from build123d import *

# Parameters (mm, degrees)
SKETCH1_R           = 3.175
BOSS_EXTRUDE1_DEPTH = 6.096
CUT_EXTRUDE1_DEPTH  = 8.636
SKETCH4_W           = 6.223
SKETCH4_H           = 7.62
CUT_EXTRUDE2_DEPTH  = 81.243500547
SKETCH5_R           = 1.651
CUT_EXTRUDE4_DEPTH  = 6.096


with BuildPart() as part:
    # Sketch1 → Boss-Extrude1 (new body)
    with BuildSketch(Plane.XY):
        Polygon((0, 0), (-38.1, 0), (-38.1, -7.62), (-31.877, -7.62), (-31.877, -15.24), (-38.1, -15.24), (-38.1, -22.86), (-31.877, -22.86), (-31.877, -30.48), (-38.1, -30.48), (-38.1, -38.1), (-31.877, -38.1), (-31.877, -45.72), (-38.1, -45.72), (-38.1, -70.358), (0, -50.8), align=None)
        with Locations(Location((-8.382, -8.382, 0), (0, 0, 180))):
            Circle(SKETCH1_R, mode=Mode.SUBTRACT)
    extrude(amount=BOSS_EXTRUDE1_DEPTH)

    # Sketch2 → Cut-Extrude1 (cut)
    with BuildSketch(Plane(origin=(0, 0, 0), x_dir=(-1, 0, 0), z_dir=(0, 0, -1))):
        Polygon((38.1, 0), (12.7, 0), (38.1, -3.81), align=None)
    extrude(amount=-CUT_EXTRUDE1_DEPTH, mode=Mode.SUBTRACT)

    # Sketch4 → Cut-Extrude2 (cut, through all)
    with BuildSketch(Plane.XY.offset(6.096)):
        with Locations((-34.9885, -57.15)):
            Rectangle(SKETCH4_W, SKETCH4_H)
    extrude(amount=-CUT_EXTRUDE2_DEPTH, mode=Mode.SUBTRACT)

    # Sketch5 → Cut-Extrude4 (cut)
    with BuildSketch(Plane(origin=(0, 0, 0), x_dir=(-1, 0, 0), z_dir=(0, 0, -1))):
        with Locations((9.318987701, -29.697415784)):
            Circle(SKETCH5_R)
    extrude(amount=-CUT_EXTRUDE4_DEPTH, mode=Mode.SUBTRACT)


solid = part.part
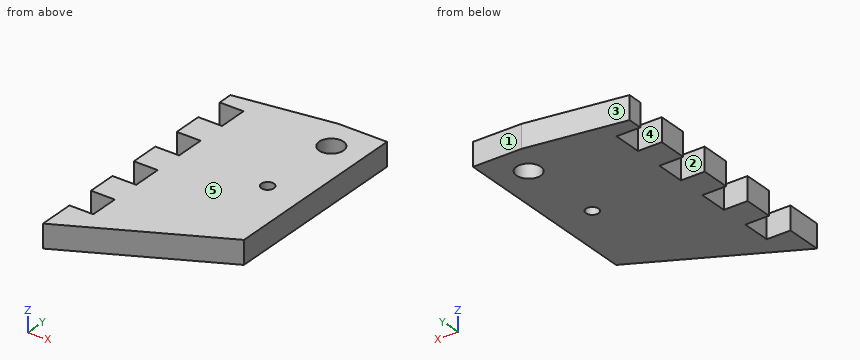
Input: part model. Units: mm. Frame: model coordinates. Face numbers are marked on the shaded views. A direction names the side the tool comes from. Give positions to 0.01 mm unless a question says otherwise; leave off trailing zeros. Write each loop counter-clockwise with the first axis right and the second up, starting at its lowest first coordinate (ties: lowest second). Pieces come first, ordered by that corner, then holes. Notation, with made-up numbers: M 35,65.25 L 70,65.25 A18 ccw 70,90.25 Z; hole C 47.5,27.5 d3. An arc over 180 degrees is marked long. Write item = value, one per line. Start each with the question number.
1) Cut plane C-C on y = -39. Return the cut outline in (x, z), then the cut area to 3 significant figures.
2) Cut plane B-B on z = 3.75. Return the cut outline in (x, y) (3 decimals).
3) Cut plane D-D on x = -3. Return the cut outline in (y, z).
4) Cut plane A-A on x = -7. Return the cut outline in (y, z), then the cut area to 3 significant figures.
5) Reachability of the marked faces 1 and 2 from +Z, -Z, +X, -X, +Y, -Y: full face, straight path, thin tool, end or side. Return the list, or none.
6) First-contact query: pin 1 Ø1.8 at (y, z) = (-28.5, 2.5) entering from -X; pin 2 Ø1.5 at (x, z) = (-22, 4.5) entering from -Y; pin 3 Ø3 at (x, z) = (-36, 3.5) entering from +Y. Flat tips, straight axial feed; report the tip coordinate or a pass-through.
7) Draft query along Y for the marked faces 3, 4 and 5. Return one class per face: +Y half, -Y half, draft (parallel to the pull), parting line (faces both ways), or undercut.
8) Material intervals for line 1 along Y through (x, z) = (-33, 0.5) (3 decimals); line 2 along Y through (x, z) = (-32, 3) (3 decimals); line 3 along X through (y, z) = (-42, 1), sorted ascending. Write a range as [from, to].
Solved:
q1.outline = M -31.88,0 L 0,0 L 0,6.1 L -31.88,6.1 Z
q1.area = 194 mm2
q2.outline = M -38.1,-70.358 L 0,-50.8 L 0,0 L -12.7,0 L -38.1,-3.81 L -38.1,-7.62 L -31.877,-7.62 L -31.877,-15.24 L -38.1,-15.24 L -38.1,-22.86 L -31.877,-22.86 L -31.877,-30.48 L -38.1,-30.48 L -38.1,-38.1 L -31.877,-38.1 L -31.877,-45.72 L -38.1,-45.72 L -38.1,-53.34 L -31.877,-53.34 L -31.877,-60.96 L -38.1,-60.96 Z; hole C -8.382,-8.382 d6.35; hole C -9.319,-29.697 d3.302
q3.outline = M -52.34,0 L 0,0 L 0,6.1 L -52.34,6.1 Z
q4.outline = M -54.39,0 L -11.24,0 L -11.24,6.1 L -54.39,6.1 Z; M -5.52,0 L 0,0 L 0,6.1 L -5.52,6.1 Z
q4.area = 297 mm2
q5.face_1 = +Z, -Z, +X, -X, +Y
q5.face_2 = +Z, -Z, -X
q6.pin_1 = -31.88
q6.pin_2 = -62.48
q6.pin_3 = -3.27
q7.face_3 = +Y half
q7.face_4 = undercut
q7.face_5 = draft
q8.line_1 = [-67.74, -60.96], [-53.34, -45.72], [-38.1, -30.48], [-22.86, -15.24], [-7.62, -3.045]
q8.line_2 = [-67.227, -60.96], [-53.34, -45.72], [-38.1, -30.48], [-22.86, -15.24], [-7.62, -2.895]
q8.line_3 = [-31.88, 0]
